from build123d import *

# Parameters (mm, degrees)
CUT_EXTRUDE1_DEPTH      = 34
CUT_EXTRUDE1_DEPTH_BACK = 34
CUT_EXTRUDE2_DEPTH      = 34.0000001
CUT_EXTRUDE2_DEPTH_BACK = 34.0000001


with BuildPart() as part:
    # Sketch1 → Revolve1 (revolve)
    with BuildSketch(Plane.XY, mode=Mode.PRIVATE) as revolve1_sk:
        Polygon((-11, 0), (-22, 0), (-33, 41), (-24.048780488, 41), (-16, 11), (-11, 11), align=None)
    revolve(revolve1_sk.sketch.rotate(Axis((0, 0, 0), (0, 1, 0)), 270), axis=Axis((0, 0, 0), (0, 1, 0)))  # turned: the seam where the file's is

    # Sketch2 → Cut-Extrude1 (cut, two sides)
    with BuildSketch(Plane.XY) as cut_extrude1_sk:
        with BuildLine():
            Line((-5, 41), (5, 41))
            ThreePointArc((5, 41), (0, 36), (-5, 41))
        make_face()
    extrude(amount=CUT_EXTRUDE1_DEPTH, mode=Mode.SUBTRACT)
    extrude(cut_extrude1_sk.sketch, amount=-CUT_EXTRUDE1_DEPTH_BACK, mode=Mode.SUBTRACT)

    # Sketch3 → Cut-Extrude2 (cut, two sides)
    with BuildSketch(Plane(origin=(0, 0, 0), x_dir=(0, 0, -1), z_dir=(1, 0, 0))) as cut_extrude2_sk:
        with BuildLine():
            Line((-5, 41), (5, 41))
            ThreePointArc((5, 41), (0, 36), (-5, 41))
        make_face()
    extrude(amount=CUT_EXTRUDE2_DEPTH, mode=Mode.SUBTRACT)
    extrude(cut_extrude2_sk.sketch, amount=-CUT_EXTRUDE2_DEPTH_BACK, mode=Mode.SUBTRACT)


solid = part.part
Can you work these out from the model? Positions are in its coordinate system, mm. Give positions to 0.01 mm unless a question says otherwise; leave off trailing zeros. Write each loop counter-clockwise with the first axis right and the second up, starting at its lowest first coordinate (ties: lowest second). Pieces come first, ordered by that corner, then holes. Notation, with made-up numbers: (25.5, 46) -> (68.5, 46) arc R28 ccw to (68.5, 75) -> close; hole circle Ø5 at (19, 37). An arc over 180 degrees is marked (long way). Answer as a JSON object with one key per item and string values. Group by question number.
Item 1: Suppose I cut it at D-D (y = 14.5). Please give me the cut outline in (x, z), plus the area to 3 significant figures.
Item 2: Suppose I cut it at A-A (x = 0). Please give me the cut outline in (y, z).
Item 3: I'm going to push flat-ended pins straight in: P1, Ø10, axis at y = 12.5, z = 16, coming from the -X side; P2, Ø12, axis at y = 16.5, z = -8, coming from the +X side; P3, Ø2, axis at x = 26, y = 5, coming from the +Z side; P4, Ø4, axis at y = 22.5, z = 25.5, coming from the -X side. Where does each tip first touch, or does it pass through?
Item 4: Suppose I cut it at C-C (y = 23). Please give me the cut outline in (x, z), plus the area to 3 significant figures.
Item 5: We'd pull the mould along X, two halves only. Please class faces 1 (the face through (3, 11, 11)), 2 (the face through (9.626, 11.676, -23.216)), 3 (the face through (-19, 41, -19)), 4 (the face through (0, 36, -28)): +X half, -X half, draft (parallel to the pull), parting line (faces both ways), or undercut.
Item 6: Please list where these lines run through material, in increasing order: line 1 (X direction, y = 13, z = 1); line 2 (X direction, y = 25, z = -4.5); line 3 (Z direction, x = -7, y = 33). Write a range as [from, to].
Item 7: Suppose I cut it at B-B (z = 0). Please give me the cut outline in (x, y), plus the area to 3 significant figures.
Findings:
{
 "1": {"outline": "circle Ø51.78 at (0, 0); hole circle Ø33.88 at (0, 0)", "area": "1,200 mm²"},
 "2": {"outline": "(0, -22) -> (36, -31.66) -> (36, -22.71) -> (11, -16) -> (11, -11) -> (0, -11) -> close; (0, 11) -> (11, 11) -> (11, 16) -> (36, 22.71) -> (36, 31.66) -> (0, 22) -> close"},
 "3": {"P1": "stops at x = -23.26", "P2": "stops at x = 27.37", "P3": "passes through", "P4": "stops at x = -15.44"},
 "4": {"outline": "circle Ø56.34 at (0, 0); hole circle Ø38.44 at (0, 0)", "area": "1,330 mm²"},
 "5": {"face 1": "undercut", "face 2": "parting line", "face 3": "draft", "face 4": "undercut"},
 "6": {"line 1": "x = [-25.47, -16.51], [16.51, 25.47]", "line 2": "x = [-28.35, -19.24], [19.24, 28.35]", "line 3": "z = [-30.05, -20.75], [20.75, 30.05]"},
 "7": {"outline": "(-31.66, 36) -> (-22, 0) -> (-11, 0) -> (-11, 11) -> (-16, 11) -> (-22.71, 36) -> close; (11, 0) -> (22, 0) -> (31.66, 36) -> (22.71, 36) -> (16, 11) -> (11, 11) -> close", "area": "722 mm²"}
}
